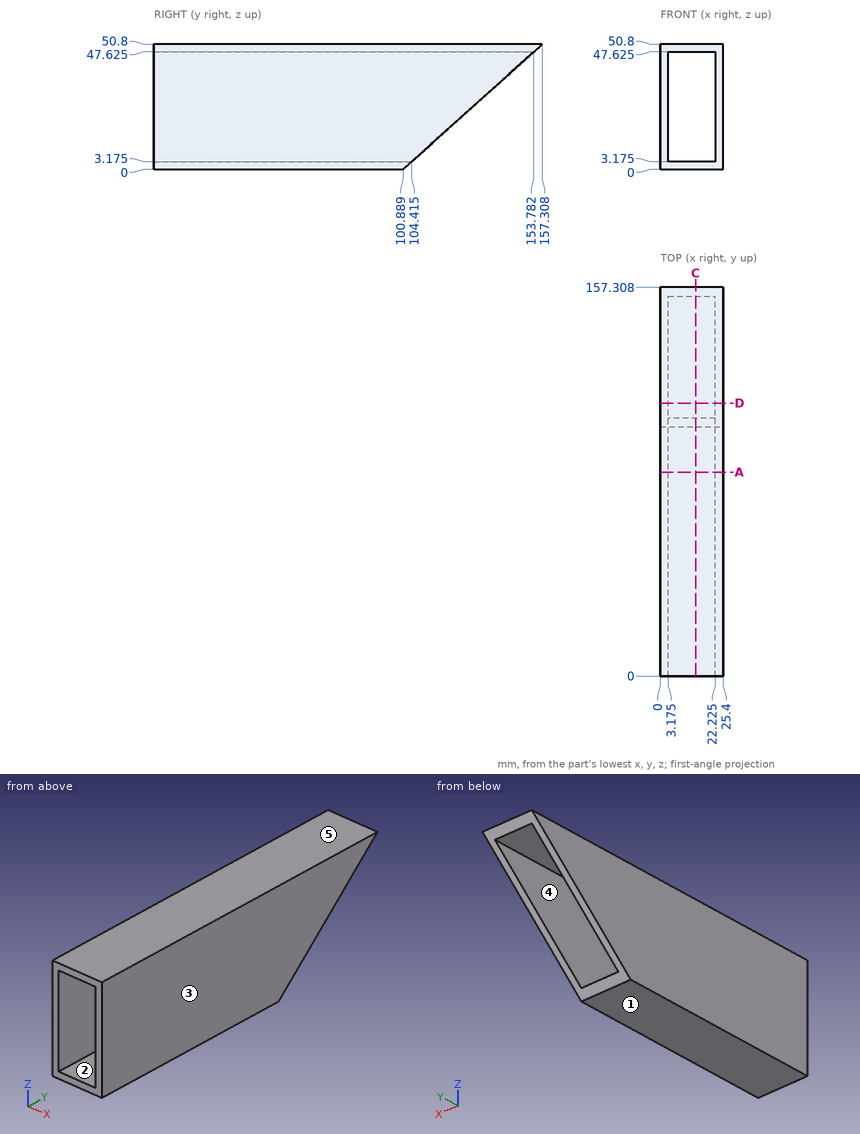
Source: three-view drawing plus pictorial views. Frame: mm from the lowest corner of the part. A direction names the side the tool comes from. Coordinates: 2 decimals unless noted, no trailing zeros. Order: outer loops, then holes, each group sorted by start corner. A loop starts at its lowest first (then second) coordinate and runs counter-clockwise, first axis right, second up. Notation, with made-up numbers: M -0.75,-17 L 40.25,-17 A28 cw 40.25,22 Z; hole C 69,39.25 d7. An arc over 180 degrees is marked long. Write each question's results on one line, items separated by ' | '. Start each with the question number.
1. Section C-C, the plane x = 14.25. Return the cut outline in (y, z) (1 decimal).
2. Reachability of the marked faces 1 and 2 from +Z, -Z, +X, -X, +Y, -Y: full face, straight path, thin tool, end or side. Return the list, or none.
3. Material intervals for L1, parallel to Z at x = 19, y = 68 (1 decimal); L2, parallel to X at y = 121.5, z = 40.5 (1 decimal); L3, parallel to Z at x = 15, y = 108 (1 decimal), sorted ascending.
4. Draft query along X for the marked faces 3, 4 and 5. Return one class per face: +X half, -X half, draft (parallel to the pull), parting line (faces both ways), or undercut.
5. Section D-D, the plane y = 110.5. Return the cut outline in (x, z) (1 decimal), then the cut area to 3 significant figures.
6. Section A-A, the plane y = 82.5. Return the cut outline in (x, z) (1 decimal).
7. Pin query (flat end, axial travel): pin 1 (2 mm diameter, centred on y = 132.5, z = 45, fed in from -X); pin 2 (12 mm diameter, centred on x = 11.5, y = 112, fed in from -Z) (3 decimals); pin 3 (10 mm diameter, centred on x = 18.5, z = 29, fed in from +Y). Return the tip coordinate at first contact, or that it passes through.
Solution:
1) outline: M 0,0 L 100.9,0 L 104.4,3.2 L 0,3.2 Z; M 0,47.6 L 153.8,47.6 L 157.3,50.8 L 0,50.8 Z
2) face 1: -Z, +X, -X, +Y, -Y | face 2: +Y, -Y
3) L1: 0 to 3.2, 47.6 to 50.8 | L2: 0 to 3.2, 22.2 to 25.4 | L3: 47.6 to 50.8
4) face 3: +X half | face 4: undercut | face 5: draft
5) outline: M 0,8.7 L 3.2,8.7 L 3.2,47.6 L 22.2,47.6 L 22.2,8.7 L 25.4,8.7 L 25.4,50.8 L 0,50.8 Z | area: 328 mm²
6) outline: M 0,0 L 25.4,0 L 25.4,50.8 L 0,50.8 Z; hole M 3.2,3.2 L 22.2,3.2 L 22.2,47.6 L 3.2,47.6 Z
7) pin 1: x = 0 | pin 2: z = 47.625 | pin 3: y = 136.8
